```python
from build123d import *


with BuildPart() as f1:
    # F0 (on Front) → F1 (revolve)
    with BuildSketch(Plane.XZ):
        with BuildLine():
            ThreePointArc((-2.5, 19.1022348606), (-14.7285015996, 13.3239396782), (-21, 1.3408993961))
            Line((-21, 1.3408993961), (-21, 0))
            Line((-21, 0), (-21, -1.4155078679))
            Line((-21, -1.4155078679), (-20, -1.4155078679))
            Line((-20, -1.4155078679), (-20, -1.276968047))
            Line((-20, -1.276968047), (-19.7798779008, -1.1605625712))
            ThreePointArc((-19.7798779008, -1.1605625712), (-19.7215120339, -1.1053626098), (-19.7, -1.0279620765))
            Line((-19.7, -1.0279620765), (-19.7, -0.8797861519))
            ThreePointArc((-19.7, -0.8797861519), (-19.7236004385, -0.7990201266), (-19.7869753447, -0.7436689494))
            Line((-19.7869753447, -0.7436689494), (-20, -0.6450347927))
            Line((-20, -0.6450347927), (-19.9719204218, 0.7546835851))
            Line((-19.9719204218, 0.7546835851), (-19.5714847863, 0.7546835851))
            ThreePointArc((-19.5714847863, 0.7546835851), (-14.2355631855, 11.6969304474), (-3.5, 17.4373580286))
            Line((-3.5, 17.4373580286), (-3.5, 17.5909579977))
            Line((-3.5, 17.5909579977), (-2.5, 17.5909579977))
            Line((-2.5, 17.5909579977), (-2.5, 19.1022348606))
        make_face()
        with BuildLine():
            Line((-21, 0), (-21, 1.3408993961))
            ThreePointArc((-21, 1.3408993961), (-21.096111691, 0.6718079569), (-21.1709106225, 0))
            Line((-21.1709106225, 0), (-21, 0))
        make_face()
        with BuildLine():
            Line((-21, -1.4155078679), (-21, 0))
            Line((-21, 0), (-21.1709106225, 0))
            ThreePointArc((-21.1709106225, 0), (-21.2263950777, -0.7070254877), (-21.2582742561, -1.4155078679))
            Line((-21.2582742561, -1.4155078679), (-21, -1.4155078679))
        make_face()
        with BuildLine():
            ThreePointArc((-3.5, 17.4373580286), (-3.0009828786, 17.5205569636), (-2.5, 17.5909579977))
            Line((-2.5, 17.5909579977), (-3.5, 17.5909579977))
            Line((-3.5, 17.5909579977), (-3.5, 17.4373580286))
        make_face()
        with BuildLine():
            Line((-2.5, 14.7757632658), (-2.5, 17.5909579977))
            ThreePointArc((-2.5, 17.5909579977), (-3.0009828786, 17.5205569636), (-3.5, 17.4373580286))
            Line((-3.5, 17.4373580286), (-3.5, 13.0909579977))
            Line((-3.5, 13.0909579977), (-2.5, 13.0909579977))
            Line((-2.5, 13.0909579977), (-2.5, 14.7757632658))
        make_face()
    revolve(axis=Axis((0, 0, 4.2133438401), (0, 0, 1)))


solid = f1.part
```
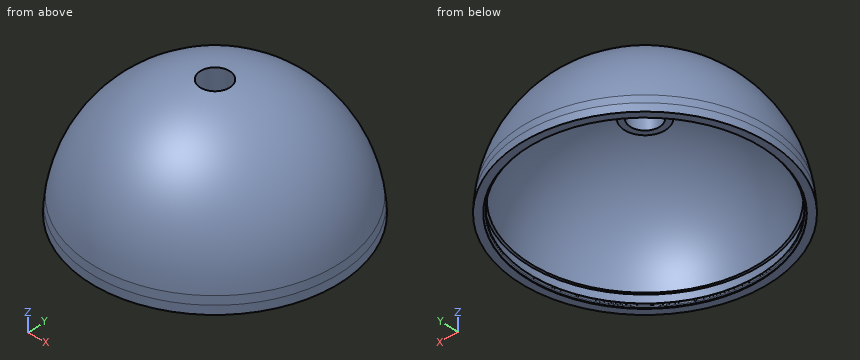
Check sheet for the modelled part. Datum: model origin and axes. Units: mm. Round coordinates to 2 decimals unless told otherwise and drop trailing zeros. Loops run counter-clockwise (first coordinate to the right, second up) from the corner with the lowest first, then second, coordinate; pieces in that order, holes last. Notation, with made-up numbers: (29.5, 86.5) - (74.5, 86.5) arc R13 ccw to (74.5, 102.5) - close; hole circle Ø4 at (15, -39). An arc over 180 degrees is marked (long way). Write item = value, one per line. Start each with the question number.
Q1. Section check A-A (y = 0). Record the boundary of the cut face in (x, z).
Q2. Thickness scan on L1, parallel to X at y = 0, z = -1.3; L2, parallel to Y at x = -14.5, z = 7; L3, parallel to X at y = 9, z = 0.5. Record the ranges inside material, lowest first.
Q3. Depth check by flat-ended pin: P1, Ø2, axis at x = 5, z = 6.5, coming from the +Y side; P2, Ø3, axis at y = 7.5, z = 1, coming from the +X side; P3, Ø5, axis at x = 6.5, z = 12.5, coming from the -Y side. Enter the tip coordinate at first touch or a pass-through.
Q4. Section check D-D (z = 7.5). Record the boundary of the cut face in (x, y), plus the area to 3 significant figures.
Q5. Section check C-C (z = 15). Record the boundary of the cut face in (x, y).
Derived:
q1.outline = (-21.26, -1.42) - (-20, -1.42) - (-20, -1.28) - (-19.78, -1.16) arc R0.15 ccw to (-19.7, -1.03) - (-19.7, -0.88) arc R0.15 ccw to (-19.79, -0.74) - (-20, -0.65) - (-19.97, 0.75) - (-19.57, 0.75) arc R19.77 cw to (-3.5, 17.44) - (-3.5, 13.09) - (-2.5, 13.09) - (-2.5, 19.1) arc R21.27 ccw to start; (2.5, 13.09) - (3.5, 13.09) - (3.5, 17.44) arc R19.77 cw to (19.57, 0.75) - (19.97, 0.75) - (20, -0.65) - (19.79, -0.74) arc R0.15 ccw to (19.7, -0.88) - (19.7, -1.03) arc R0.15 ccw to (19.78, -1.16) - (20, -1.28) - (20, -1.42) - (21.26, -1.42) arc R21.27 ccw to (2.5, 19.1) - close
q2.L1 = -21.25 to -20, 20 to 21.25
q2.L2 = -12.68 to -9.96, 9.96 to 12.68
q2.L3 = -19.1 to -17.83, 17.83 to 19.1
q3.P1 = 19.33
q3.P2 = 20.22
q3.P3 = -16.51
q4.outline = circle Ø38.04 at (0, 0); hole circle Ø34.65 at (0, 0)
q4.area = 193 mm^2
q5.outline = circle Ø25.51 at (0, 0); circle Ø7 at (0, 0); hole circle Ø20.11 at (0, 0); hole circle Ø5 at (0, 0)
